For this review, take the finished solid that the model builds, in its own axes (mm). Face numbers are marked on the shaded views. Give positions to 0.01 mm unless a question says otherwise; leave off trailing zeros. Order: outer loops, then holes, each group sorted by start corner. A loop starts at its lowest first (then second) coordinate and runs counter-clockwise, first axis right, second up. Notation, with made-up numbers: (-33, 61) -> (25, 61) arc R24 cw to (25, 89) -> close; hole circle Ø7 at (45, -14). An arc over 180 degrees is marked (long way). Return JSON: item names as keys, results as strings. Group by question number.
1) Insertion check: P1, Ø4, axis at y = 4.5, z = 6, coming from the -X side; P2, Ø3, axis at x = -33.34, y = -19.25, coming from the +Z side; P3, Ø1.5, axis at x = 12, z = 6.5, coming from the -Y side; P4, Ø5, axis at x = -17.5, z = 5.5, coming from the -Y side. Each pin has a flat end and moves straight along its axis. Give the tip position at first contact, or say it passes through.
2) The part is to be moulded in two halves that separate along X. For the marked faces 1, 2 and 3, say which applies: released by +X, released by -X, zero draft, split by the parting line, or undercut.
3) Add section C-C (z = 4.25). Give the boundary of the cut face in (x, y), then the cut area to 3 significant figures.
4) Add section A-A (x = 0). Give the boundary of the cut face in (y, z).
5) To check wall thickness, follow line 1 along Y through (x, z) = (0, 5.5); line 2 along Y through (x, z) = (0, 10.05); line 3 along X through (y, z) = (1, 2.5). State the ranges of each line that lie inside material, in increasing order.
6) Add section B-B (y = 0). Give the boundary of the cut face in (x, z).
7) Add section D-D (x = 31). Give the boundary of the cut face in (y, z), then the cut area to 3 significant figures.
from build123d import *

# Parameters (mm, degrees)
SKETCH_1_R         = 43
SKETCH_1_R_2       = 36
EXTRUDE_1_DEPTH    = 9
SKETCH_2_R         = 43
SKETCH_2_R_2       = 33
EXTRUDE_2_DEPTH    = 3
HOLE_WIZARD_M3_1_D = 2.5


with BuildPart() as part:
    # 草图1 → 凸台-拉伸1 (new body)
    with BuildSketch(Plane.XY):
        Circle(SKETCH_1_R)
        Circle(SKETCH_1_R_2, mode=Mode.SUBTRACT)
    extrude(amount=EXTRUDE_1_DEPTH)

    # 草图2 → 凸台-拉伸2 (add)
    with BuildSketch(Plane.XY.offset(9)):
        Circle(SKETCH_2_R)
        Circle(SKETCH_2_R_2, mode=Mode.SUBTRACT)
    extrude(amount=EXTRUDE_2_DEPTH)

    # M3 螺纹孔1 (through all)
    with Locations(Plane(origin=(-33.341978046, 19.25, 0), x_dir=(-1, 0, 0), z_dir=(0, 0, -1))):
        with Locations((0, 0), (-33.341978046, 19.25), (-66.683956092, 0), (-66.683956092, -38.5), (-33.341978046, -57.75), (0, -38.5)):
            Hole(HOLE_WIZARD_M3_1_D / 2)


solid = part.part
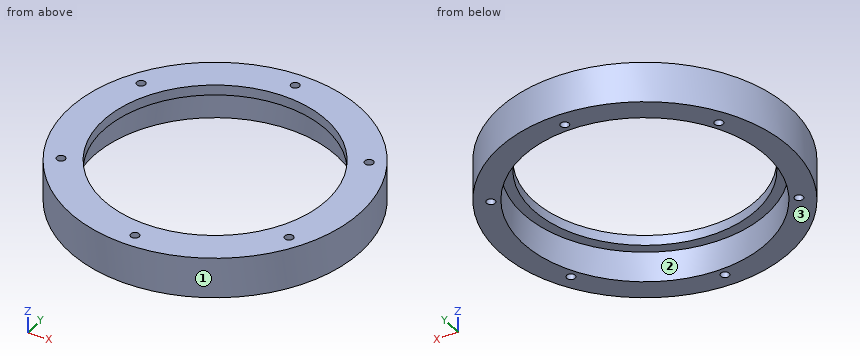
Evaluation:
{
 "1": {"P1": "x = -42.93", "P2": "z = 12", "P3": "y = -41.5", "P4": "y = -40.3"},
 "2": {"face 1": "split by the parting line", "face 2": "undercut", "face 3": "zero draft"},
 "3": {"outline": "circle Ø86 at (0, 0); hole circle Ø72 at (0, 0); hole circle Ø2.5 at (-33.34, -19.25); hole circle Ø2.5 at (-33.34, 19.25); hole circle Ø2.5 at (0, -38.5); hole circle Ø2.5 at (0, 38.5); hole circle Ø2.5 at (33.34, -19.25); hole circle Ø2.5 at (33.34, 19.25)", "area": "1,710 mm^2"},
 "4": {"outline": "(-43, 0) -> (-39.75, 0) -> (-39.75, 12) -> (-43, 12) -> close; (-37.25, 0) -> (-36, 0) -> (-36, 9) -> (-33, 9) -> (-33, 12) -> (-37.25, 12) -> close; (33, 9) -> (36, 9) -> (36, 0) -> (37.25, 0) -> (37.25, 12) -> (33, 12) -> close; (39.75, 0) -> (43, 0) -> (43, 12) -> (39.75, 12) -> close"},
 "5": {"line 1": "-43 to -39.75, -37.25 to -36, 36 to 37.25, 39.75 to 43", "line 2": "-43 to -39.75, -37.25 to -33, 33 to 37.25, 39.75 to 43", "line 3": "-42.99 to -35.99, 35.99 to 42.99"},
 "6": {"outline": "(-43, 0) -> (-36, 0) -> (-36, 9) -> (-33, 9) -> (-33, 12) -> (-43, 12) -> close; (33, 9) -> (36, 9) -> (36, 0) -> (43, 0) -> (43, 12) -> (33, 12) -> close"},
 "7": {"outline": "(-29.8, 0) -> (-18.3, 0) -> (-18.3, 9) -> (-11.31, 9) -> (-11.31, 12) -> (-29.8, 12) -> close; (11.31, 9) -> (18.3, 9) -> (18.3, 0) -> (29.8, 0) -> (29.8, 12) -> (11.31, 12) -> close", "area": "318 mm^2"}
}
